Answer from the drawing. Dimensions are ordinates in mm from the lowest x, y and z of the part. A direction names the side the tool comes from. Coordinates: 2 decimals unless noted, no trailing zeros. Order: outer loops, then holes, each group sorted by start corner. A loop starts at its lowest first (then second) coordinate and runs counter-clockwise, first axis right, second up. Notation, with made-up numbers: (-24, 48) -> (2, 48) arc R8 ccw to (2, 58) -> close; hole circle Ø4 at (-13, -36). An arc over 180 degrees is marked (long way). Answer as a JSON object with one key per item and string values. Group by question number.
1) Section D-D on x = 7.5 is taken. Determine the outline of the cut face in (y, z), and give its area (3 significant figures).
2) Given pin 1 (4 mm diameter, centred on x = 12.5, z = 12.5, fed in from -Y); pin 2 (1.5 mm diameter, centred on y = 1, z = 16.5, fed in from -X); pin 3 (4 mm diameter, centred on x = 6.5, z = 13, fed in from +Y); pin 4 (1.5 mm diameter, centred on x = 18, y = 7.5, fed in from +Z), each flat-ended and moving along its own axis, determine where each tip first touches the part or whether it passes through.
3) A tool of negligible diameter and unlimited length cuts with its end or side. For the marked faces 5, 6 and 7, from which of +Z, -Z, +X, -X, +Y, -Y can it reach the whole face along a straight path? Write none if from no direction.
4) Consider L1, parallel to Z at x = 12.5, y = 2.85; L2, parallel to X at y = 6.75, z = 12.75; L3, parallel to Y at x = 5.75, z = 19.5. Determine where each line is inside the solid, lowest interval first.
5) Determine the mould class of the marked faces 1, 2, 3 and 4 for opening direction X: released by +X, released by -X, zero draft, split by the parting line, or undercut.
6) Section B-B on y = 5.5 is taken. Determine the outline of the cut face in (x, z).
7) Section C-C on z = 2.5 is taken. Determine the outline of the cut face in (x, y).
8) Section A-A on x = 12.5 is taken. Determine the outline of the cut face in (y, z), and give its area (3 significant figures).
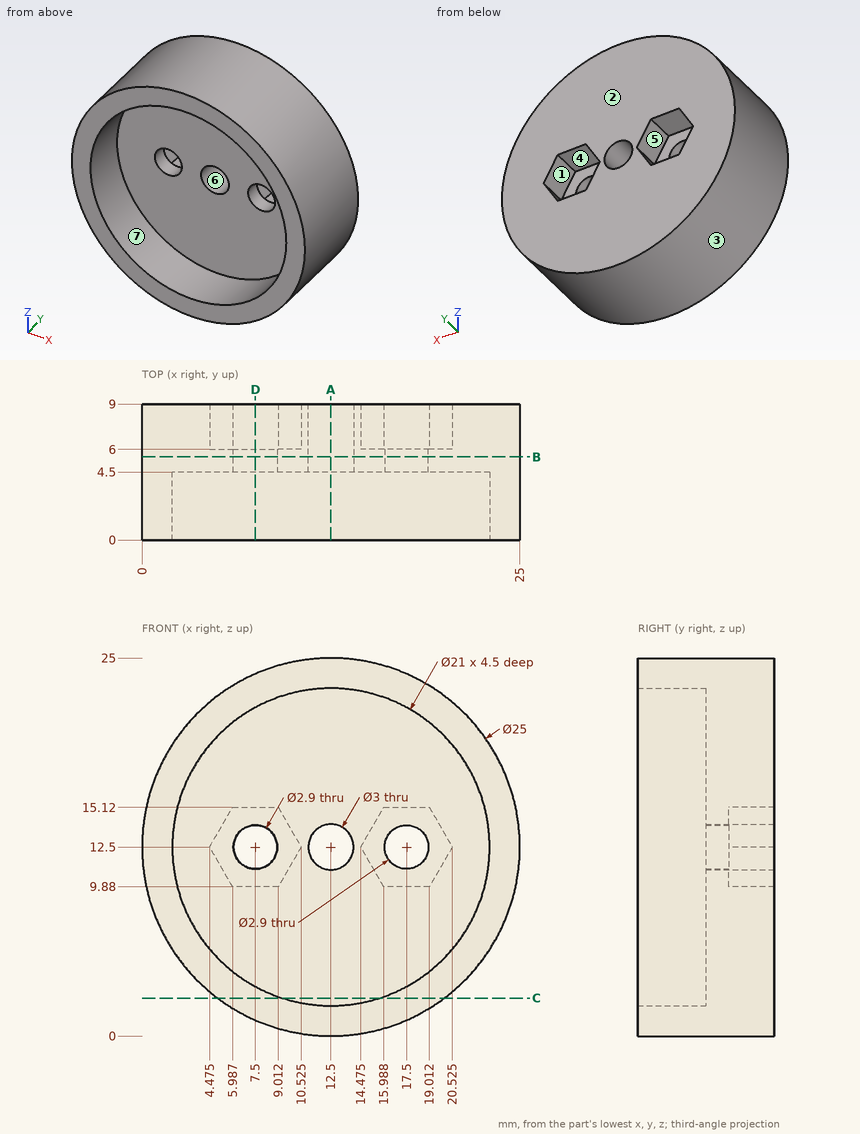
Worked answers:
{
 "1": {"outline": "(0, 1.04) -> (9, 1.04) -> (9, 9.88) -> (6, 9.88) -> (6, 11.05) -> (4.5, 11.05) -> (4.5, 3.27) -> (0, 3.27) -> close; (0, 21.73) -> (4.5, 21.73) -> (4.5, 13.95) -> (6, 13.95) -> (6, 15.12) -> (9, 15.12) -> (9, 23.96) -> (0, 23.96) -> close", "area": "103 mm²"},
 "2": {"pin 1": "stops at y = 4.5", "pin 2": "stops at x = 0.43", "pin 3": "stops at y = 9", "pin 4": "stops at z = 24.06"},
 "3": {"face 5": "+Y", "face 6": "+Y, -Y", "face 7": "-Y"},
 "4": {"L1": "z = 0 to 2, 23 to 25", "L2": "x = 0 to 4.62, 10.38 to 11.02, 13.98 to 14.62, 20.38 to 25", "L3": "y = 4.5 to 9"},
 "5": {"face 1": "undercut", "face 2": "zero draft", "face 3": "split by the parting line", "face 4": "undercut"},
 "6": {"outline": "circle Ø25 at (12.5, 12.5); hole circle Ø2.9 at (7.5, 12.5); hole circle Ø3 at (12.5, 12.5); hole circle Ø2.9 at (17.5, 12.5)"},
 "7": {"outline": "(5, 0) -> (9.3, 0) -> (9.3, 4.5) -> (15.7, 4.5) -> (15.7, 0) -> (20, 0) -> (20, 9) -> (5, 9) -> close"},
 "8": {"outline": "(0, 0) -> (9, 0) -> (9, 11) -> (4.5, 11) -> (4.5, 2) -> (0, 2) -> close; (0, 23) -> (4.5, 23) -> (4.5, 14) -> (9, 14) -> (9, 25) -> (0, 25) -> close", "area": "117 mm²"}
}
